```python
from build123d import *

# Parameters (mm, degrees)
ESQUISSE1_R                  = 28
BOSS_EXTRU_1_DEPTH           = 5
ESQUISSE2_R                  = 4
BOSS_EXTRU_2_DEPTH           = 10
ESQUISSE3_R                  = 2.1
ENL_V_MAT_EXTRU_1_DEPTH      = 43.343830719
ESQUISSE4_R                  = 2
ESQUISSE5_R                  = 6
ESQUISSE5_R_2                = 4
BOSS_EXTRU_3_DEPTH           = 6
ENL_V_MAT_EXTRU_2_REACH      = 44.344
ENL_V_MAT_EXTRU_2_END_RADIUS = 6
ESQUISSE6_R                  = 1.5


with BuildPart() as part:
    # Esquisse1 → Boss.-Extru.1 (new body)
    with BuildSketch(Plane.XY):
        Circle(ESQUISSE1_R)
    extrude(amount=BOSS_EXTRU_1_DEPTH)

    # Esquisse2 → Boss.-Extru.2 (add)
    with BuildSketch(Plane.XY.offset(5)):
        Circle(ESQUISSE2_R)
    extrude(amount=BOSS_EXTRU_2_DEPTH)

    # Esquisse3 → Enlèv. mat.-Extru.1 (cut, through all)
    with BuildSketch(Plane.XY.offset(15)):
        Circle(ESQUISSE3_R)
    extrude(amount=-ENL_V_MAT_EXTRU_1_DEPTH, mode=Mode.SUBTRACT)

    # Esquisse4 → Enlèvement de matière-Révolution1 (revolve, cut)
    with BuildSketch(Plane(origin=(0, 0, 0), x_dir=(0, 0, -1), z_dir=(1, 0, 0)), mode=Mode.PRIVATE) as enl_vement_de_mati_re_r_volution1_sk:
        with Locations((-2.5, 28)):
            Circle(ESQUISSE4_R)
    revolve(enl_vement_de_mati_re_r_volution1_sk.sketch.rotate(Axis((0, 0, 0), (0, 0, 1)), 90), axis=Axis((0, 0, 0), (0, 0, 1)), mode=Mode.SUBTRACT)

    # Esquisse5 → Boss.-Extru.3 (add)
    with BuildSketch(Plane.XY.offset(5)):
        Circle(ESQUISSE5_R)
        Circle(ESQUISSE5_R_2, mode=Mode.SUBTRACT)
    extrude(amount=BOSS_EXTRU_3_DEPTH)

    # Enlèv. mat.-Extru.2: up to this cylinder (the profile starts inside it)
    enl_v_mat_extru_2_end = Plane(origin=(0, 0, 8), z_dir=(0, 0, -1)) * Cylinder(ENL_V_MAT_EXTRU_2_END_RADIUS, 101.688, mode=Mode.PRIVATE)
    # Esquisse6 → Enlèv. mat.-Extru.2 (cut, up to the surface)
    with BuildSketch(Plane(origin=(0, 0, 0), x_dir=(1, 0, 0), z_dir=(0, 1, 0)), mode=Mode.PRIVATE) as enl_v_mat_extru_2_sk1:
        with Locations(Location((0, -8, 0), (0, 0, 90))):
            Circle(ESQUISSE6_R)
    enl_v_mat_extru_2_tool1 = extrude(enl_v_mat_extru_2_sk1.sketch, amount=ENL_V_MAT_EXTRU_2_REACH, mode=Mode.PRIVATE) & enl_v_mat_extru_2_end
    add(enl_v_mat_extru_2_tool1.solids().sort_by_distance((0, 0, 8))[0], mode=Mode.SUBTRACT)


solid = part.part
```
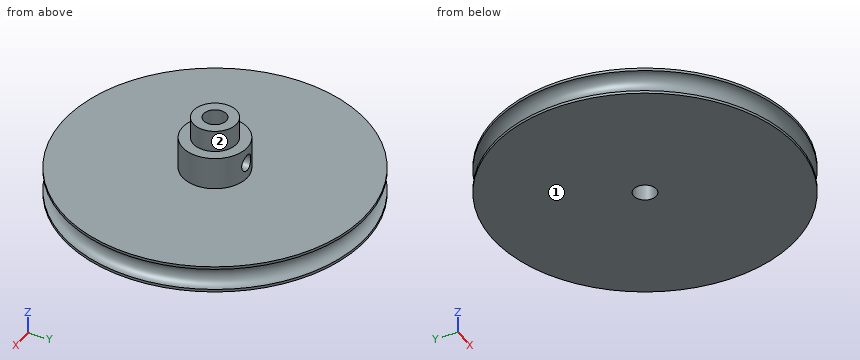
Verification items for the finished model (mm, model axes). Face numbers are marked on the shaded views. A direction names the side the tool comes from. Round coordinates to 2 decimals unless told otherwise and drop trailing zeros. Order: outer loops, then holes, each group sorted by start corner. A loop starts at its lowest first (then second) coordinate and runs counter-clockwise, first axis right, second up. Notation, with made-up numbers: (52.25, -34) -> (88.25, -34) arc R32 cw to (88.25, 4) -> close; hole circle Ø9 at (35.25, 47). An arc over 180 degrees is marked (long way). Put each result on its own line as item: value. Start each with the question number.
(1) Material ranges on line 1 along Z through (x, y) = (-18.5, 15); line 2 along X through (y, z) = (4.25, 8); line 3 along X through (y, z) = (4.55, 8), recorded low to high.
(2) Section check B-B (z = 12.25). Enter the section's corners in (x, y).
(3) Tool access check on the marked faces 1 and 2. Record the directions out of +Z, -Z, +X, -X, +Y, -Y that give a thin tool (end or side, any length) a straight path to the whole face; none if there is none.
(4) Section check D-D (z = 2). Enter the section's corners in (x, y), then the cut area to 3 significant figures.
(5) Depth check by flat-ended pin: pin 1 Ø3.5 at (x, z) = (0, 8) entering from +Y; pin 2 Ø2 at (y, z) = (15, 4.5) entering from -X. Enter the tip coordinate at first touch or a pass-through.
(6) Section check A-A (x = 0). Enter the section's corners in (y, z).
(7) Section check C-C (z = 8.25). Enter the section's corners in (x, y).
Completed:
1. line 1: z = 0 to 5
1. line 2: x = -4.24 to -1.5, 1.5 to 4.24
1. line 3: x = -3.91 to -1.5, 1.5 to 3.91
2. outline: circle Ø8 at (0, 0); hole circle Ø4.2 at (0, 0)
3. face 1: -Z, +X, -X, +Y, -Y
3. face 2: +Z
4. outline: circle Ø52.13 at (0, 0); hole circle Ø4.2 at (0, 0)
4. area: 2,120 mm2
5. pin 1: stops at y = 6
5. pin 2: stops at x = -24.25
6. outline: (-28, 0) -> (-2.1, 0) -> (-2.1, 15) -> (-4, 15) -> (-4, 11) -> (-6, 11) -> (-6, 5) -> (-28, 5) -> (-28, 4.5) arc R2 cw to (-28, 0.5) -> close; (2.1, 0) -> (28, 0) -> (28, 0.5) arc R2 cw to (28, 4.5) -> (28, 5) -> (6, 5) -> (6, 6.5) -> (2.1, 6.5) -> close; (2.1, 9.5) -> (6, 9.5) -> (6, 11) -> (4, 11) -> (4, 15) -> (2.1, 15) -> close
7. outline: (-1.48, 1.49) -> (-1.48, 5.81) arc R6 ccw (long way) to (1.48, 5.81) -> (1.48, 1.49) arc R2.1 cw (long way) to start
